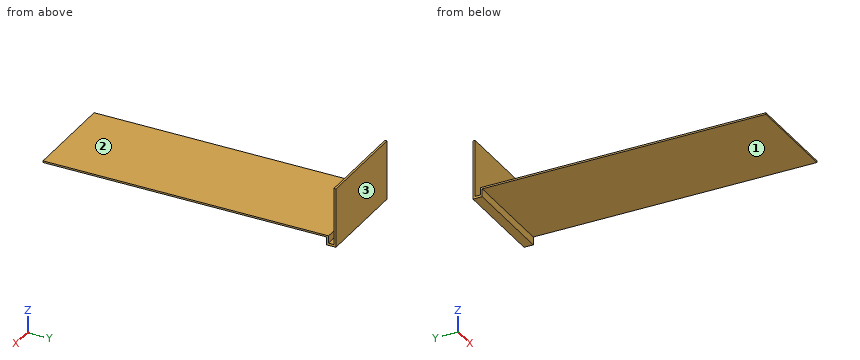
from build123d import *

# Parameters (mm, degrees)
F0_W     = 58
F0_H     = 170
F1_DEPTH = 1
F3_DEPTH = 58


with BuildPart() as f1:
    # F0 (on Top) → F1 (new body)
    with BuildSketch(Plane.XY):
        Rectangle(F0_W, F0_H)
    extrude(amount=F1_DEPTH)

    # F2 (on face) → F3 (join, through all)
    with BuildSketch(Plane.YZ.offset(29)):
        Polygon((86.109489, 1), (85, 1), (85, -4.806199), (86.109489, -4.806199), (90.539046, -4.806199), (90.539046, -3.463339), (90.539046, 30.797509), (89.292906, 30.797509), (89.292906, -3.463339), (86.109489, -3.463339), align=None)
    extrude(amount=-F3_DEPTH)


solid = f1.part
Here's how the part is built. I have some questions about the finished solid (model axes, mm). Face numbers are marked on the shaded views. A direction names the side the tool comes from. Coordinates: 2 decimals unless noted, no trailing zeros. Order: outer loops, then holes, each group sorted by start corner. A loop starts at its lowest first (then second) coordinate and runs counter-clockwise, first axis right, second up. Notation, with made-up numbers: (70, -28) - (91, -28) arc R32 cw to (91, 2) - close; hole circle Ø3 at (-31, 39). An arc over 180 degrees is marked (long way). Use CSV: the item, a comma, the result in double quotes. Start each with the question number.
1. I'm going to push flat-ended pins straight in: pin 1 (12 mm diameter, centred on x = 13, y = 47.5, fed in from -Z); pin 2 (2.5 mm diameter, centred on x = 6, z = -2, fed in from -Y); pin 3 (4 mm diameter, centred on x = 12.5, y = -56, fed in from +Z); pin 4 (3.5 mm diameter, centred on x = 1.5, y = 88, fed in from +Z). Where does each tip first touch, or does it pass through?
2. For the marked faces 1, 2 and 3, which set-ups out of +Z, -Z, +X, -X, +Y, -Y let a thin tool reach every point of the face, with its end or its side?
3. Please list where these lines run through material, in increasing order: line 1 (Y direction, x = -8.5, z = -1.5); line 2 (Y direction, x = -11.5, z = 0.5); line 3 (Y direction, x = 12.5, z = 22.5). Write a range as from..to.
4. Suppose I cut it at A-A on x = 20.5. List the corners of the cut face in (y, z) for me.
5. Suppose I cut it at C-C on y = -73.5. List the corners of the cut face in (x, z) for me, then the cut area to 3 significant figures.
6. Suppose I cut it at B-B on z = 20. List the corners of the cut face in (x, y) for me, then the cut area to 3 significant figures.
Output:
1,pin 1,"stops at z = 0"
1,pin 2,"stops at y = 85"
1,pin 3,"stops at z = 1"
1,pin 4,"stops at z = 30.8"
2,face 1,"-Z, +X, -X, -Y"
2,face 2,"+Z, +X, -X, -Y"
2,face 3,"+Z, -Z, +X, -X, +Y"
3,line 1,"y = 85..86.11, 89.29..90.54"
3,line 2,"y = -85..86.11, 89.29..90.54"
3,line 3,"y = 89.29..90.54"
4,outline,"(-85, 0) - (85, 0) - (85, -4.81) - (90.54, -4.81) - (90.54, 30.8) - (89.29, 30.8) - (89.29, -3.46) - (86.11, -3.46) - (86.11, 1) - (-85, 1) - close"
5,outline,"(-29, 0) - (29, 0) - (29, 1) - (-29, 1) - close"
5,area,"58.0 mm2"
6,outline,"(-29, 89.29) - (29, 89.29) - (29, 90.54) - (-29, 90.54) - close"
6,area,"72.3 mm2"
